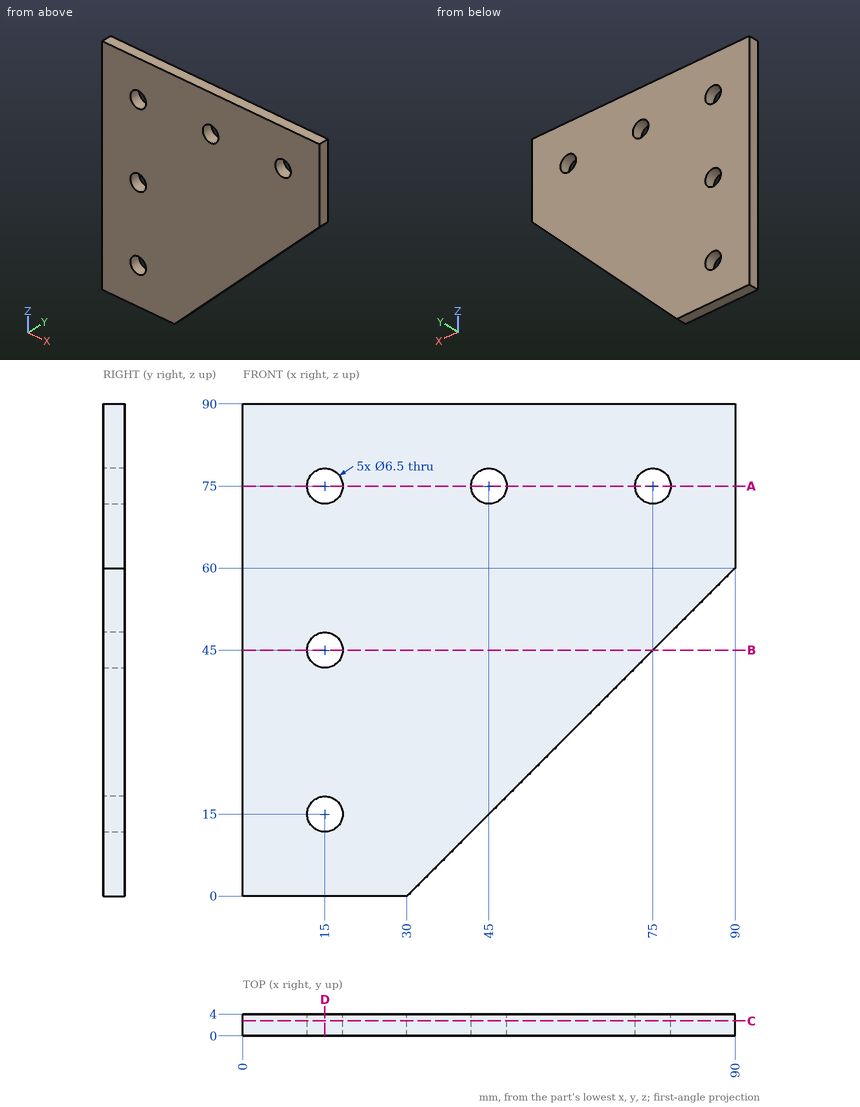
Could you check a few things on this drawing? It's one solid part, dimensions in mm from its lowest x, y, z. Round coordinates to 2 decimals unless told otherwise and drop trailing zeros. Write each loop counter-clockwise with the first axis right and the second up, starting at its lowest first coordinate (ties: lowest second). Pieces come first, ordered by that corner, then holes.
Q1. If we section it at D-D on x = 15: Write out the boundary of the cut face in (y, z), plus the area to 3 significant figures.
Q2. If we section it at B-B on z = 45: Write out the boundary of the cut face in (x, y), plus the area to 3 significant figures.
Q3. Please list where these lines run through material, in increasing order: probe 1 along X at (y, z) = (1.45, 75); probe 2 along X at (y, z) = (1.35, 45); probe 3 along Z at (x, y) = (73, 3.55).
Q4. If we section it at C-C on y = 2.75: Write out the boundary of the cut face in (x, z), plus the area to 3 significant figures.
Q5. Will this pin go through, and if not, where does the flat tip stop? P1, Ø4, axis at x = 15, z = 75, coming from the -Y side.
Q6. If we section it at A-A on z = 75: Write out the boundary of the cut face in (x, y), plus the area to 3 significant figures.
Answer below:
1. outline: (0, 0) - (4, 0) - (4, 11.75) - (0, 11.75) - close; (0, 18.25) - (4, 18.25) - (4, 41.75) - (0, 41.75) - close; (0, 48.25) - (4, 48.25) - (4, 71.75) - (0, 71.75) - close; (0, 78.25) - (4, 78.25) - (4, 90) - (0, 90) - close
1. area: 282 mm2
2. outline: (0, 0) - (11.75, 0) - (11.75, 4) - (0, 4) - close; (18.25, 0) - (75, 0) - (75, 4) - (18.25, 4) - close
2. area: 274 mm2
3. probe 1: x = 0 to 11.75, 18.25 to 41.75, 48.25 to 71.75, 78.25 to 90
3. probe 2: x = 0 to 11.75, 18.25 to 75
3. probe 3: z = 43 to 72.44, 77.56 to 90
4. outline: (0, 0) - (30, 0) - (90, 60) - (90, 90) - (0, 90) - close; hole circle Ø6.5 at (15, 15); hole circle Ø6.5 at (15, 45); hole circle Ø6.5 at (15, 75); hole circle Ø6.5 at (45, 75); hole circle Ø6.5 at (75, 75)
4. area: 6,130 mm2
5. P1: passes through
6. outline: (0, 0) - (11.75, 0) - (11.75, 4) - (0, 4) - close; (18.25, 0) - (41.75, 0) - (41.75, 4) - (18.25, 4) - close; (48.25, 0) - (71.75, 0) - (71.75, 4) - (48.25, 4) - close; (78.25, 0) - (90, 0) - (90, 4) - (78.25, 4) - close
6. area: 282 mm2
